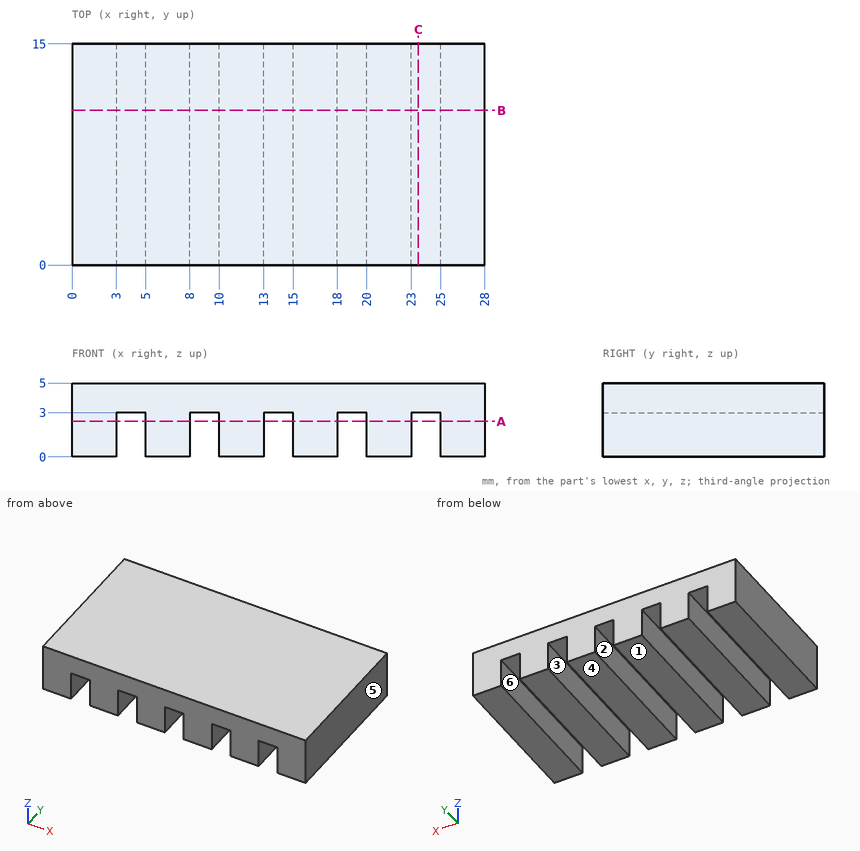
Can you work these out from the drawing? Everything is in mm from the part's minimum corner. A direction names the side the tool comes from. Give positions to 0.01 mm unless a question says otherwise; leave off trailing zeros. Loops run counter-clockwise (first coordinate to the right, second up) from the corner with the lowest first, then second, coordinate; pieces in that order, holes last. Notation, with made-up numbers: M 55.25,-13 L 91.25,-13 A12 ccw 91.25,9 Z; hole C 62,68.25 d10. An arc over 180 degrees is marked long. Use CSV: the item, a comma, the result in double quotes. Start each with the question number.
1. On a 3-axis mill with a long thin cutter (end or side, diameter ignored), from which of +Z, -Z, +X, -X, +Y, -Y can I reach the whole of each face in a straight line? I mean the marked faces 1 and 2. Say none if no direction works.
2. For P1, Ø1, axis at x = 12, y = 4, coming from the -Z side; P2, Ø1, axis at x = 9, y = 5, coming from the -Z side, each with a flat end and sliding along its axis, tell me the tip position at first contact or that it passes through.
3. Imagine slicing it at C-C, the plane x = 23.5. Write out the boundary of the cut face in (y, z).
4. If I drill on L1, parallel to X at y = 5.25, z = 1.8; L2, parallel to Z at x = 19.5, y = 12.25, over which ranges is the centre line in solid material (lowest first)?
5. Imagine slicing it at A-A, the plane z = 2.4. Write out the boundary of the cut face in (x, y).
6. If we mould it in two halves opening along X, with no side actions, what happens to the marked faces 3, 4, 5 and 6? For each: released by +X, released by -X, zero draft, split by the parting line, or undercut.
7. Imagine slicing it at B-B, the plane y = 10.5. Write out the boundary of the cut face in (x, z).
Response values:
1,face 1,"-Z, +X, -X, +Y, -Y"
1,face 2,"-Z, +Y, -Y"
2,P1,"z = 0"
2,P2,"z = 3"
3,outline,"M 0,3 L 15,3 L 15,5 L 0,5 Z"
4,L1,"0 to 3, 5 to 8, 10 to 13, 15 to 18, 20 to 23, 25 to 28"
4,L2,"3 to 5"
5,outline,"M 0,0 L 3,0 L 3,15 L 0,15 Z; M 5,0 L 8,0 L 8,15 L 5,15 Z; M 10,0 L 13,0 L 13,15 L 10,15 Z; M 15,0 L 18,0 L 18,15 L 15,15 Z; M 20,0 L 23,0 L 23,15 L 20,15 Z; M 25,0 L 28,0 L 28,15 L 25,15 Z"
6,face 3,"undercut"
6,face 4,"zero draft"
6,face 5,"released by +X"
6,face 6,"undercut"
7,outline,"M 0,0 L 3,0 L 3,3 L 5,3 L 5,0 L 8,0 L 8,3 L 10,3 L 10,0 L 13,0 L 13,3 L 15,3 L 15,0 L 18,0 L 18,3 L 20,3 L 20,0 L 23,0 L 23,3 L 25,3 L 25,0 L 28,0 L 28,5 L 0,5 Z"
